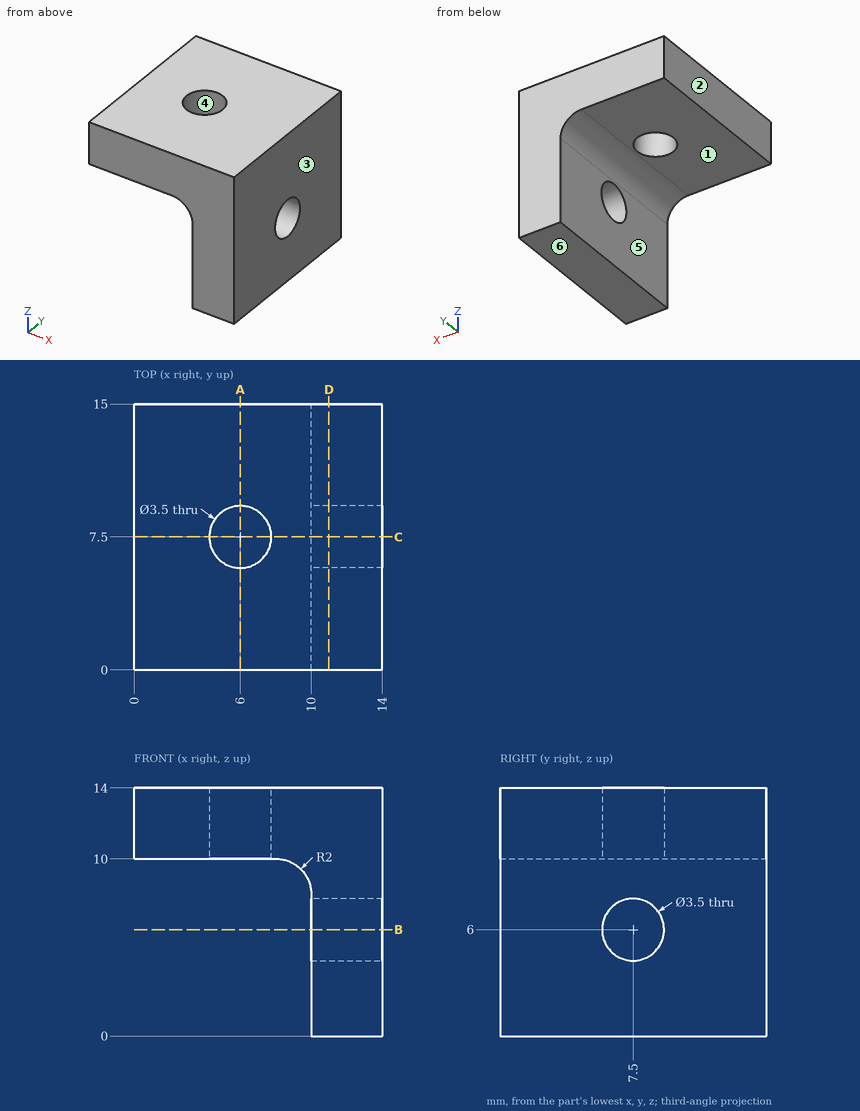
Print and shaded views of the part. All mm, measured from the part's lowest x, y and z. A direction names the side the tool comes from. Round coordinates to 2 decimals unless told otherwise and drop trailing zeros. Loops run counter-clockwise (first coordinate to the right, second up) from the corner with the lowest first, then second, coordinate; pieces in that order, holes last. Notation, with made-up numbers: (16.5, -18.75) -> (51.5, -18.75) arc R20 ccw to (51.5, -11.75) -> close; hole circle Ø6 at (55.25, 60.25). An arc over 180 degrees is marked (long way). Use CSV: the item, a comma, the result in double quotes. Start each with the question number.
1) Cut at D-D, the plane x = 11. Write the cut outline in (y, z).
2) Pull direction X, two halves, no side cores. Call the marked faces 1, 2, 3 and 4: +X half, -X half, draft (parallel to the pull), parting line (faces both ways), or undercut.
3) Cut at A-A, the plane x = 6. Write the cut outline in (y, z).
4) Drop flat-ended pins along their axis: P1, Ø8, axis at x = 5, y = 4.5, coming from the -Z side; P2, Ø2, axis at y = 7.5, z = 6, coming from the +X side; P3, Ø5.5, axis at x = 6, y = 7.5, coming from the -Z side. Give the stop position or say it passes through.
5) Cut at C-C, the plane y = 7.5. Write the cut outline in (x, z).
6) Wall check: L1, parallel to Y at x = 6, z = 12.65; L2, parallel to X at y = 1.5, z = 2. Give the ranges that are in metal, low to high. Write a range as [from, to].
7) Cut at B-B, the plane z = 6. Write the cut outline in (x, y).
8) Which spindle directions (+Z, -Z, +X, -X, +Y, -Y) get a long thin tool onto all of the face, cutting with end or side? Do the marked faces 5 and 6. Say none if no direction does.
Determined:
1,outline,"(0, 0) -> (15, 0) -> (15, 14) -> (0, 14) -> close; hole circle Ø3.5 at (7.5, 6)"
2,face 1,"draft"
2,face 2,"-X half"
2,face 3,"+X half"
2,face 4,"undercut"
3,outline,"(0, 10) -> (5.75, 10) -> (5.75, 14) -> (0, 14) -> close; (9.25, 10) -> (15, 10) -> (15, 14) -> (9.25, 14) -> close"
4,P1,"stops at z = 9.73"
4,P2,"passes through"
4,P3,"stops at z = 9.85"
5,outline,"(0, 10) -> (4.25, 10) -> (4.25, 14) -> (0, 14) -> close; (7.75, 10) -> (8, 10) arc R2 cw to (10, 8) -> (10, 7.75) -> (14, 7.75) -> (14, 14) -> (7.75, 14) -> close; (10, 0) -> (14, 0) -> (14, 4.25) -> (10, 4.25) -> close"
6,L1,"y = [0, 5.75], [9.25, 15]"
6,L2,"x = [10, 14]"
7,outline,"(10, 0) -> (14, 0) -> (14, 5.75) -> (10, 5.75) -> close; (10, 9.25) -> (14, 9.25) -> (14, 15) -> (10, 15) -> close"
8,face 5,"-Z, -X, +Y, -Y"
8,face 6,"-Z, +X, -X, +Y, -Y"
